Work out the finished part from the listing and answer in its coordinate system (mm). A direction names the side the tool comes from. Coordinates: 2 decimals unless noted, no trailing zeros. Order: outer loops, then holes, each group sorted by start corner. A loop starts at its lowest first (then second) coordinate and runs counter-clockwise, first axis right, second up.
1. The part is cut by section C-C, the plane x = 0. Give the vertices of the cut face in (y, z).
2. Find the intervals of material crossed by probe 1 along X at (y, z) = (28.5, 0.7); probe 2 along Y at (x, z) = (113, 0.35); probe 3 along Y at (x, z) = (13.5, 0.5), in increasing order.
3. A flat-ended cylindrical pin translates along its axis: pin 1 Ø3 at (x, y) = (0.5, -35) entering from -Z. Find the tip coordinate at first contact, or state that the pin passes through.
4. The part is cut by section D-D, the plane y = -70. Give the vertices of the cut face in (x, z), then the cut area to 3 significant figures.
5. The part is cut by section A-A, the plane z = 0.65. Give the vertices of the cut face in (x, y).
6. A tool of negligible diameter and unlimited length cuts with its end or side. For faces 1 (the flat face through (-2, -36, 0)), 2 (the flat face through (68.287, 39.425, 0.493)), from which of +Z, -Z, +X, -X, +Y, -Y can it reach the whole face along a straight path? Write none if from no direction.
7. The part is cut by section B-B, the plane y = 17.5. Give the vertices of the cut face in (x, z).
Autodesk Inventor part; units mm, degrees
ref_plane "YZ Plane" through (0, 0, 0) normal (1, 0, 0) x (0, 1, 0)
ref_plane "XZ Plane" through (0, 0, 0) normal (0, 1, 0) x (-1, 0, 0)
ref_plane "XY Plane" through (0, 0, 0) normal (0, 0, 1) x (1, 0, 0)
sketch "Sketch1" plane through (0, 0, 0) normal (0, 0, 1) x (1, 0, 0)
  arc A0 (-131.9823, 76.2) -> (131.9823, 76.2) centre (0, 0) ccw
  line L0 (6.35, 3.6662) -> (131.9823, 76.2)
  line L1 (0, 0) -> (152.4, 0) construction
  line L2 (-6.35, 3.6662) -> (-85.8668, 49.5752)
  line L3 (0, 0) -> (99.1504, 0) construction
  line L4 (-85.8668, 49.5752) -> (-131.9823, 76.2)
  line L5 (0, 0) -> (6.35, 0)
  line L6 (6.35, 0) -> (6.35, 3.6662)
  line L7 (0, 0) -> (-6.35, 0)
  line L8 (-6.35, 0) -> (-6.35, 3.6662)
  dimension "d0" = 304.8
  dimension "d1" = 30
  dimension "d2" = 150
  dimension "d3" = 6.35
  dimension "d4" = 6.35
extrude "Extrusion1" add sketch "Sketch1" along normal blind 1
properties part number "view2"
Geometry says:
1. outline: (-152.4, 0) - (0, 0) - (0, 1) - (-152.4, 1) - close
2. probe 1: x = -149.71 to -49.36, 49.36 to 149.71
2. probe 2: y = -102.26 to 65.24
2. probe 3: y = -151.8 to 7.79
3. pin 1: stops at z = 0
4. outline: (-135.37, 0) - (135.37, 0) - (135.37, 1) - (-135.37, 1) - close
4. area: 271 mm2
5. outline: (-131.98, 76.2) arc R152.4 ccw (long way) to (131.98, 76.2) - (6.35, 3.67) - (6.35, 0) - (-6.35, 0) - (-6.35, 3.67) - (-85.87, 49.58) - close
6. face 1: -Z, +X, -X, +Y, -Y
6. face 2: +Z, -Z, +Y
7. outline: (-151.39, 0) - (-30.31, 0) - (-30.31, 1) - (-151.39, 1) - close; (30.31, 0) - (151.39, 0) - (151.39, 1) - (30.31, 1) - close
